from build123d import *

# Parameters (mm, degrees)
SKETCH1_W             = 25.4
SKETCH1_H             = 9.525
BOSS_EXTRUDE1_DEPTH   = 13.97
CUT_EXTRUDE1_DEPTH    = 1.50114
F_4_40_TAPPED_HOLE1_D = 2.2606
SKETCH5_R             = 2.6543
CUT_EXTRUDE2_DEPTH    = 7.62
FILLET1_R             = 1.905


with BuildPart() as part:
    # Sketch1 → Boss-Extrude1 (new body)
    with BuildSketch(Plane.XY):
        Rectangle(SKETCH1_W, SKETCH1_H)
    extrude(amount=BOSS_EXTRUDE1_DEPTH)

    # Sketch2 → Cut-Extrude1 (cut)
    with BuildSketch(Plane.XY.offset(13.97)):
        Polygon((10.6, 3.525), (12.7, 3.525), (12.7, 4.7625), (-12.7, 4.7625), (-12.681617083, 3.525), (-10.6, 3.525), (-8.9, 1.825), (-8.9, -3.175), (8.9, -3.175), (8.9, 1.825), align=None)
        Polygon((12.7, 3.398), (12.7, 3.525), (10.6, 3.525), (8.9, 1.825), (8.9, -3.175), (-8.9, -3.175), (-8.9, 1.825), (-10.6, 3.525), (-12.681617083, 3.525), (-12.7, 4.7625), (-12.7, 3.398), (-10.652605122, 3.398), (-9.027, 1.772394878), (-9.027, -3.302), (9.027, -3.302), (9.027, 1.772394878), (10.652605122, 3.398), align=None)
    extrude(amount=-CUT_EXTRUDE1_DEPTH, mode=Mode.SUBTRACT)

    # #4-40 Tapped Hole1 (through all)
    with Locations(Plane.XY.offset(12.46886)):
        with Locations((-3.2, 0.125), (3.2, 0.125)):
            Hole(F_4_40_TAPPED_HOLE1_D / 2)

    # Sketch5 → Cut-Extrude2 (cut)
    with BuildSketch(Plane.XZ.offset(4.7625)):
        with Locations(Location((-6.985, 6.985, 0), (0, 0, 270))):
            Circle(SKETCH5_R)
        with Locations(Location((6.985, 6.985, 0), (0, 0, 270))):
            Circle(SKETCH5_R)
    extrude(amount=-CUT_EXTRUDE2_DEPTH, mode=Mode.SUBTRACT)

    # Fillet1
    fillet1_edges = [part.edges().sort_by_distance(p)[0] for p in [
        (-12.7, 4.7625, 6.23443),
        (0, 4.7625, 0),
        (12.7, 4.7625, 6.23443),
    ]]
    fillet(fillet1_edges, radius=FILLET1_R)


solid = part.part
Geometry: final body of the model. Coordinates: model frame, mm. A direction names the side the tool comes from. Give positions to 0.01 mm unless a question says otherwise; leave off trailing zeros. Order: outer loops, then holes, each group sorted by start corner. A loop starts at its lowest first (then second) coordinate and runs counter-clockwise, first axis right, second up. Notation, with made-up numbers: (35.25, -23) -> (60.25, -23) arc R17 cw to (60.25, -2) -> close; hole circle Ø4 at (65, -27.75). An arc over 180 degrees is marked (long way). Put each result on its own line as item: value.
Q1. Material intervals for L1, parallel to Y at x = 3.2, z = 5.5; L2, parallel to X at y = 0, z = 8; L3, parallel to X at y = -0.25, z = 4.25, sorted ascending.
Here are the results:
L1: y = -4.76 to -1.01, 1.26 to 4.76
L2: x = -12.7 to -9.44, -4.53 to -4.32, -2.08 to 2.08, 4.32 to 4.53, 9.44 to 12.7
L3: x = -12.7 to -4.27, -2.13 to 2.13, 4.27 to 12.7
Q2. Section D-D, the plane x = 8. Return loops of the section in (y, z) (1 decimal).
Here are the results:
outline: (-4.8, 0) -> (2.9, 0) arc R1.9 ccw to (4.8, 1.9) -> (4.8, 12.5) -> (-3.3, 12.5) -> (-3.3, 14) -> (-4.8, 14) -> (-4.8, 9.4) -> (2.9, 9.4) -> (2.9, 4.5) -> (-4.8, 4.5) -> close
Q3. Section C-C, the plane y = -1.75. Return loops of the section in (x, z) (3 decimals), then the cut area to 3 significant figures.
Here are the results:
outline: (-12.7, 0) -> (12.7, 0) -> (12.7, 13.97) -> (9.027, 13.97) -> (9.027, 12.469) -> (-9.027, 12.469) -> (-9.027, 13.97) -> (-12.7, 13.97) -> close; hole circle Ø5.309 at (-6.985, 6.985); hole circle Ø5.309 at (6.985, 6.985)
area: 283 mm^2
Q4. Pin query (flat end, axial travel): pin 1 (0.5 mm diameter, centred on x = -3, z = 13, fed in from +Y); pin 2 (1 mm diameter, centred on x = -1, y = -1, fed in from -Z); pin 3 (2.5 mm diameter, centred on x = 8, z = 6.5, fed in from -Y); pin 4 (0.8 mm diameter, centred on x = -11.5, z = 13.5, fed in from +Y). Return the tip coordinate at first contact, or that it passes through.
Here are the results:
pin 1: stops at y = -3.3
pin 2: stops at z = 0
pin 3: stops at y = 2.86
pin 4: stops at y = 3.4
Q5. Reachability of faces 1 (the face through (0, -4.762, 7)), 2 (the face through (9.828, 2.574, 13.23)), 3 (the face through (-7, 2.858, 7)), 4 (the face through (0, -1, 0)), 5 (the face through (12, 3.398, 13)) from +Z, -Z, +X, -X, +Y, -Y: full face, straight path, thin tool, end or side. Return the list, or none.
Here are the results:
face 1: +Z, -Z, +X, -X, -Y
face 2: +Z, +Y
face 3: -Y
face 4: -Z, +X, -X, +Y, -Y
face 5: +Z, +X, -X, +Y
Q6. Draft query along X for faces 6 (the face through (-12, 3.398, 13)), 7 (the face through (-9.851, 2.597, 13.23)), 8 (the face through (-9.027, -1, 13)), 9 (the face through (12.127, 4.219, 7.083)). Return one class per face: released by +X, released by -X, zero draft, split by the parting line, or undercut.
Here are the results:
face 6: zero draft
face 7: undercut
face 8: undercut
face 9: released by +X
Q7. Section B-B, the plane z = 3.75. Return loops of the section in (x, y) (1 decimal), then the cut area to 3 significant figures.
Here are the results:
outline: (-12.7, -4.8) -> (12.7, -4.8) -> (12.7, 2.9) arc R1.9 ccw to (10.8, 4.8) -> (-10.8, 4.8) arc R1.9 ccw to (-12.7, 2.9) -> close; hole circle Ø2.3 at (-3.2, 0.1); hole circle Ø2.3 at (3.2, 0.1)
area: 232 mm^2
Q8. Section A-A, the plane x = -3.2. Return loops of the section in (y, z) (1 decimal), then the cut area to 3 significant figures.
Here are the results:
outline: (-4.8, 0) -> (-1, 0) -> (-1, 12.5) -> (-3.3, 12.5) -> (-3.3, 14) -> (-4.8, 14) -> close; (1.3, 0) -> (2.9, 0) arc R1.9 ccw to (4.8, 1.9) -> (4.8, 12.5) -> (1.3, 12.5) -> close
area: 92.0 mm^2
